from build123d import *

# Parameters (mm, degrees)
CUT_EXTRUDE1_DEPTH      = 13.280472369
CUT_EXTRUDE1_DEPTH_BACK = 13.280472369
CUT_EXTRUDE2_DEPTH      = 13.280472369
CUT_EXTRUDE2_DEPTH_BACK = 13.280472369
FILLET2_R               = 0.254
SKETCH5_R               = 1.211430269
CUT_EXTRUDE3_DEPTH      = 10


with BuildPart() as part:
    # Sketch2 → Revolve1 (revolve)
    with BuildSketch(Plane(origin=(0, 0, 0), x_dir=(0, 0, -1), z_dir=(1, 0, 0)), mode=Mode.PRIVATE) as revolve1_sk:
        with BuildLine():
            Line((-10.9, 0), (-10.9, 0.8))
            Line((-10.9, 0.8), (-1, 0.8))
            ThreePointArc((-1, 0.8), (-0.811032662, 2.442902614), (-0.254, 4))
            Line((-0.254, 4), (0, 4))
            Line((0, 4), (0, 2))
            Line((0, 2), (6.6, 2))
            Line((6.6, 2), (6.6, 1.5))
            add(Edge.make_bspline(
                [(8.1, 0), (8.1, 4.430500874), (6.6, 1.5)],
                knots=[4.71238898, 4.71238898, 4.71238898, 7.005919555, 7.005919555, 7.005919555], degree=2, weights=[1, 0.411437828, 1]))
            Line((8.1, 0), (6.6, 0))
            Line((6.6, 0), (-10.9, 0))
        make_face()
    revolve(revolve1_sk.sketch.rotate(Axis((0, 0, 10.9), (0, 0, -1)), 90), axis=Axis((0, 0, 10.9), (0, 0, -1)))

    # Sketch3 → Cut-Extrude1 (cut, two sides: drawn at the far end of the back side and taken through both)
    with BuildSketch(Plane(origin=(0, 0, 0), x_dir=(1, 0, 0), z_dir=(0, 1, 0)).offset(-CUT_EXTRUDE1_DEPTH_BACK)):
        Polygon((0, -10.9), (1.0032, -9.592604306), (1.0032, -11.408), (-1.0032, -11.408), (-1.0032, -9.592604306), align=None)
    extrude(amount=CUT_EXTRUDE1_DEPTH + CUT_EXTRUDE1_DEPTH_BACK, mode=Mode.SUBTRACT)

    # Sketch4 → Cut-Extrude2 (cut, two sides: drawn at the far end of the back side and taken through both)
    with BuildSketch(Plane(origin=(0, 0, 0), x_dir=(0, 0, -1), z_dir=(1, 0, 0)).offset(-CUT_EXTRUDE2_DEPTH_BACK)):
        Polygon((-11.154, 0), (-9.846, 1.308), (-11.408, 1.308), (-11.408, -1.308), (-9.846, -1.308), align=None)
    extrude(amount=CUT_EXTRUDE2_DEPTH + CUT_EXTRUDE2_DEPTH_BACK, mode=Mode.SUBTRACT)

    # Fillet2
    fillet2_edges = [part.edges().sort_by_distance(p)[0] for p in [
        (-2, 0, 0),
    ]]
    fillet(fillet2_edges, radius=FILLET2_R)

    # Sketch5 → Cut-Extrude3 (cut)
    with BuildSketch(Plane(origin=(0, 0, 1.1), x_dir=(-1, 0, 0), z_dir=(0, 0, -1))):
        Circle(SKETCH5_R)
    extrude(amount=-CUT_EXTRUDE3_DEPTH, mode=Mode.SUBTRACT)


solid = part.part
Input: part model. Units: mm. Frame: model coordinates. A direction names the side the tool comes from. Coordinates: 2 decimals unless noted, no trailing zeros. Loops run counter-clockwise (first coordinate to the right, second up) from the corner with the lowest first, then second, coordinate; pieces in that order, holes last.
Q1. Cut plane A-A (z = -5.25). Output: boundary loops of the cut face in (x, y).
Q2. Material intervals for line 1 (Y direction, x = 0, z = -3.75); line 2 (X direction, y = 1.5, z = -3); line 3 (Y direction, x = 0.5, z = -1.5), sorted ascending.
Q3. Contact query for flat-ended pins moving along their axis: pin 1 (2 mm diameter, centred on x = -1.5, z = -2, fed in from -Y); pin 2 (4 mm diameter, centred on x = -2, z = -5, fed in from +Y); pin 3 (2 mm diameter, centred on x = -2.5, z = -2, fed in from +Y). Output: stop coordinate, or through.
Q4. Set-up query: faces 1 (the face through (0, 0, 1.1)), 2 (the face through (2, 2, 0)). Return all of +Z, -Z, +X, -X, +Y, -Y with unobstructed straight access to the full face (end or side cutting, diameter ignored); none if empty.
Working result:
1. outline: circle Ø4 at (0, 0)
2. line 1: y = -2 to 2
2. line 2: x = -1.32 to 1.32
2. line 3: y = -1.94 to 1.94
3. pin 1: stops at y = -1.94
3. pin 2: stops at y = 2
3. pin 3: stops at y = 1.32
4. face 1: +Z, +X, -X, +Y, -Y
4. face 2: -Z
